Check sheet for the modelled part. Datum: model origin and axes. Units: mm. Give positions to 0.01 mm unless a question says otherwise; leave off trailing zeros. Loops run counter-clockwise (first coordinate to the right, second up) from the corner with the lowest first, then second, coordinate; pieces in that order, holes last. Notation, with made-up numbers: M 16,20 L 28,20 A24 ccw 28,37 Z; hole C -9.75,79 d9. An arc over 180 degrees is marked long. Write each question's results on one line, items separated by ' | '. Start each with the question number.
1. Sectioned sample at A-A on y = -3. Record the cut outline in (x, z).
2. Sectioned sample at C-C on y = -200. Record the cut outline in (x, z), and give its area (3 significant figures).
3. Sectioned sample at B-B on z = 1.75. Record the cut outline in (x, y).
4. Go/stop test with flat-tipped pins: pin 1 (0.6 mm diameter, centred on y = -4, z = 4.5, fed in from +X); pin 2 (0.6 mm diameter, centred on y = -3.5, z = 4.5, fed in from -X); pin 3 (3 mm diameter, centred on x = 4, y = -140.5, fed in from +Z). Record where each tip stops, or that it passes through.
5. Material ranges on line 1 along Y through (x, z) = (7.5, 1.5); line 2 along Z through (x, y) = (2.5, -52.5); line 3 along Y through (x, z) = (4.5, 3), recorded low to high.
```python
from build123d import *

# Parameters (mm, degrees)
F1_DEPTH = 219.5
F3_DEPTH = 3.6
F6_W     = 3
F6_H     = 3
F7_ANGLE = 180
F8_R     = 1


with BuildPart() as f1:
    # F0 (on Front) → F1 (new body)
    with BuildSketch(Plane.XZ):
        Polygon((2.0784609691, 3.6), (0, 0), (9.8, 0), (7.7215390309, 3.6), align=None)
    extrude(amount=F1_DEPTH)

    # F2 (on face) → F3 (join)
    with BuildSketch(Plane(origin=(0, 0, 0), x_dir=(1, 0, 0), z_dir=(0, 0, -1))):
        with BuildLine():
            ThreePointArc((7.0931712199, 219.5), (7.3220784514, 220.0806971863), (7.4, 220.7))
            ThreePointArc((7.4, 220.7), (4.2806971863, 223.1220784514), (2.7068287801, 219.5))
            Line((2.7068287801, 219.5), (7.0931712199, 219.5))
        make_face()
    extrude(amount=-F3_DEPTH)


with BuildPart() as f4_1:
    # F4: copy of F1
    add(f1.part)

    # F6 (on face) → F7 (revolve)
    with BuildSketch(Plane.XY.offset(3.6)):
        with Locations((4.9, -1.5)):
            Rectangle(F6_W, F6_H)
    revolve(axis=Axis((4.9, -3, 3.6), (1, 0, 0)), revolution_arc=F7_ANGLE)

    # F8
    f8_edges = [f4_1.edges().sort_by_distance(p)[0] for p in [
        (6.4, -3, 6.6),
        (3.4, -3, 6.6),
    ]]
    fillet(f8_edges, radius=F8_R)


solid = f4_1.part
```
Output values:
1) outline: M 0,0 L 9.8,0 L 7.72,3.6 L 6.4,3.6 L 6.4,5.6 A1 ccw 5.4,6.6 L 4.4,6.6 A1 ccw 3.4,5.6 L 3.4,3.6 L 2.08,3.6 Z
2) outline: M 0,0 L 9.8,0 L 7.72,3.6 L 2.08,3.6 Z | area: 27.8 mm2
3) outline: M 1.01,-219.5 L 2.71,-219.5 A2.5 ccw long 7.09,-219.5 L 8.79,-219.5 L 8.79,0 L 1.01,0 Z
4) pin 1: x = 6.4 | pin 2: x = 3.4 | pin 3: z = 3.6
5) line 1: -219.5 to 0 | line 2: 0 to 3.6 | line 3: -223.17 to 0
